For this review, take the finished solid that the model builds, in its own axes (mm). A direction names the side the tool comes from. Give positions to 0.01 mm unless a question says otherwise; leave off trailing zeros. Write each loop counter-clockwise with the first axis right and the second up, starting at its lowest first coordinate (ties: lowest second). Pieces come first, ordered by that corner, then holes. Notation, with made-up numbers: (-19, -36) -> (22, -36) arc R19 cw to (22, -28) -> close; hole circle Ø3 at (13, -5). An arc over 180 degrees is marked (long way). Answer as CSV lines item,"result".
Autodesk Inventor part; units mm, degrees
ref_plane "YZ Plane" through (0, 0, 0) normal (1, 0, 0) x (0, 1, 0)
ref_plane "XZ Plane" through (0, 0, 0) normal (0, 1, 0) x (-1, 0, 0)
ref_plane "XY Plane" through (0, 0, 0) normal (0, 0, 1) x (1, 0, 0)
sketch "スケッチ1" plane through (0, 0, 0) normal (1, 0, 0) x (0, 1, 0)
  line L0 (-114.0211, -198.214) -> (-114.0211, 205.786)
  line L1 (-114.0211, 122.786) -> (139.9789, 122.786)
  line L2 (139.9789, 122.786) -> (139.9789, 107.786)
  line L3 (139.9789, 107.786) -> (-114.0211, 107.786)
  line L4 (-114.0211, 107.786) -> (-114.0211, 122.786)
  line L5 (-74.0211, 147.286) -> (134.9789, 147.286)
  line L6 (134.9789, 147.286) -> (134.9789, -139.714)
  line L7 (134.9789, -139.714) -> (-74.0211, -139.714)
  line L8 (-74.0211, -139.714) -> (-74.0211, 147.286)
  line L9 (-134.0211, -198.214) -> (-134.0211, 205.786)
  line L10 (-134.0211, 3.786) -> (-114.0211, 3.786)
  line L11 (-114.0211, 205.786) -> (-134.0211, 205.786)
  line L12 (-114.0211, -115.214) -> (139.9789, -115.214)
  line L13 (139.9789, -100.214) -> (-114.0211, -100.214)
  line L14 (139.9789, -115.214) -> (139.9789, -100.214)
  line L15 (92.4789, 157.286) -> (82.4789, 157.286)
  line L16 (82.4789, 157.286) -> (82.4789, 3.786)
  line L17 (82.4789, 3.786) -> (92.4789, 3.786)
  line L18 (92.4789, 3.786) -> (92.4789, 157.286)
  line L19 (-21.5211, 157.286) -> (-31.5211, 157.286)
  line L20 (-31.5211, 157.286) -> (-31.5211, 3.786)
  line L21 (-31.5211, 3.786) -> (-21.5211, 3.786)
  line L22 (-21.5211, 3.786) -> (-21.5211, 157.286)
  line L23 (-114.0211, 135.286) -> (-134.0211, 135.286)
  line L24 (-84.0211, 122.786) -> (-84.0211, 107.786)
  circle A0 centre (-124.0211, 115.286) radius 1.5
  circle A1 centre (-124.0211, 125.286) radius 1.5
  line L25 (-114.0211, 135.286) -> (-114.0211, 122.786)
  line L26 (-114.0211, 107.786) -> (-134.0211, 107.786)
  line L27 (-134.0211, 135.286) -> (-134.0211, 107.786)
  circle A2 centre (-104.0211, 115.286) radius 1.5
  circle A3 centre (-94.0211, 115.286) radius 1.5
  line L28 (-84.0211, 107.786) -> (-64.0211, 107.786)
  line L29 (-64.0211, 107.786) -> (-64.0211, 101.786)
  line L30 (-64.0211, 101.786) -> (-84.0211, 101.786)
  line L31 (-84.0211, 101.786) -> (-84.0211, 107.786)
  line L32 (-31.5211, 157.286) -> (-37.5211, 157.286)
  line L33 (-37.5211, 157.286) -> (-37.5211, 137.286)
  line L34 (-37.5211, 137.286) -> (-31.5211, 137.286)
  line L35 (-31.5211, 137.286) -> (-31.5211, 157.286)
  line L36 (92.4789, 157.286) -> (98.4789, 157.286)
  line L37 (98.4789, 157.286) -> (98.4789, 137.286)
  line L38 (98.4789, 137.286) -> (92.4789, 137.286)
  line L39 (92.4789, 137.286) -> (92.4789, 157.286)
  line L40 (30.4789, 147.286) -> (30.4789, -139.714)
  line L41 (134.9789, 3.786) -> (-114.0211, 3.786)
  line L42 (-114.0211, 205.786) -> (-114.0211, -198.214)
  line L43 (-84.0211, -94.214) -> (-84.0211, -100.214)
  line L44 (-64.0211, -94.214) -> (-84.0211, -94.214)
  line L45 (-64.0211, -100.214) -> (-64.0211, -94.214)
  line L46 (-84.0211, -115.214) -> (-84.0211, -100.214)
  circle A4 centre (-94.0211, -107.714) radius 1.5
  circle A5 centre (-104.0211, -107.714) radius 1.5
  circle A6 centre (-124.0211, -107.714) radius 1.5
  circle A7 centre (-124.0211, -117.714) radius 1.5
  line L47 (-114.0211, -127.714) -> (-134.0211, -127.714)
  line L48 (-114.0211, -100.214) -> (-134.0211, -100.214)
  line L49 (-37.5211, -149.714) -> (-37.5211, -129.714)
  line L50 (-31.5211, -149.714) -> (-37.5211, -149.714)
  line L51 (-21.5211, -149.714) -> (-31.5211, -149.714)
  line L52 (-31.5211, -149.714) -> (-31.5211, 3.786)
  line L53 (-21.5211, 3.786) -> (-21.5211, -149.714)
  line L54 (-37.5211, -129.714) -> (-31.5211, -129.714)
  line L55 (82.4789, -149.714) -> (82.4789, 3.786)
  line L56 (92.4789, -149.714) -> (82.4789, -149.714)
  line L57 (92.4789, -149.714) -> (98.4789, -149.714)
  line L58 (98.4789, -149.714) -> (98.4789, -129.714)
  line L59 (98.4789, -129.714) -> (92.4789, -129.714)
  line L60 (92.4789, 3.786) -> (92.4789, -149.714)
  circle A8 centre (-26.5211, 115.286) radius 1.5
  circle A9 centre (87.4789, 115.286) radius 1.5
  circle A10 centre (87.4789, -107.714) radius 1.5
  circle A11 centre (-26.5211, -107.714) radius 1.5
  line L61 (-114.0211, 122.786) -> (-114.0211, 107.786)
  line L62 (-114.0211, -100.214) -> (-114.0211, -115.214)
  point P0 (0, 0)
  point P1 (-114.0211, 3.786)
  point P2 (-114.0211, 3.786)
  point P3 (-114.0211, 107.786)
  dimension "d0" = 15
  dimension "d1" = 287
  dimension "d2" = 209
  dimension "d3" = 83
  dimension "d4" = 10
  dimension "d5" = 10
  dimension "d6" = 30
  dimension "d7" = 3
  dimension "d8" = 7.5
  dimension "d9" = 10
  dimension "d10" = 3
  dimension "d11" = 10
  dimension "d12" = 10
  dimension "d13" = 10
  dimension "d14" = 3
  dimension "d15" = 3
  dimension "d16" = 10
  dimension "d17" = 10
  dimension "d18" = 7.5
  dimension "d19" = 7.5
  dimension "d20" = 6
  dimension "d21" = 10
  dimension "d22" = 10
  dimension "d23" = 5
  dimension "d24" = 143.5
  dimension "d25" = 10
  dimension "d26" = 6
  dimension "d27" = 20
  dimension "d28" = 10
  dimension "d29" = 6
  dimension "d30" = 20
  dimension "d31" = 0
  dimension "d32" = 0
  dimension "d33" = 52
  dimension "d34" = 52
  dimension "d35" = 3
  dimension "d36" = 3
  dimension "d37" = 5
  dimension "d38" = 7.5
  dimension "d39" = 7.5
  dimension "d40" = 5
extrude "押し出し1" add sketch "スケッチ1" against normal blind 2 contours L26 L9 L23 L0 | L0 L1 L24 L3
fillet "フィレット1" radius 2 6 edges at (-1, -84.0211, 122.786) (-1, -84.0211, 107.786) (-1, -114.0211, 122.786) (-1, -114.0211, 135.286) (-1, -134.0211, 135.286) (-1, -134.0211, 107.786)
equation "\"d13\" = d9"
equation "\"d17\" = d16"
equation "\"d19\" = d18"
equation "\"d34\" = d33"
properties part number "base_weel-v2-Plate-8" material "アルミニウム 6061"
Q1. Add section C-C (z = 114.25). Write out the cut boundary in (x, y).
Answer block:
outline,"(-2, -134.02) -> (0, -134.02) -> (0, -125.11) -> (-2, -125.11) -> close; (-2, -122.94) -> (0, -122.94) -> (0, -105.11) -> (-2, -105.11) -> close; (-2, -102.94) -> (0, -102.94) -> (0, -95.11) -> (-2, -95.11) -> close; (-2, -92.94) -> (0, -92.94) -> (0, -84.02) -> (-2, -84.02) -> close"
Q2. For faces 1 (the flat face through (0, -115, 119)), 2 (the flat face through (-1, -114.021, 129)), list the 3-axis set-ups (+Z, -Z, +X, -X, +Y, -Y) from which the entire face can be reached by the end or side of a thin tool; tool diameter is ignored.
Answer block:
face 1,"+Z, -Z, +X, +Y, -Y"
face 2,"+Z, +X, -X, +Y"
Q3. To check wall thickness, follow probe 1 along Z at (x, y) = (-1.7, -94); probe 2 along Y at (x, z) = (-0.55, 127.5); probe 3 along Y at (x, z) = (-0.65, 115.5). State the ranges of each line that lie inside material, in increasing order. Write a range as [from, to].
Answer block:
probe 1,"z = [107.79, 113.79], [116.79, 122.79]"
probe 2,"y = [-134.02, -114.02]"
probe 3,"y = [-134.02, -125.51], [-122.54, -105.51], [-102.54, -95.51], [-92.54, -84.02]"
Q4. Add section D-D (z = 126). Write out the cut boundary in (x, y).
Answer block:
outline,"(-2, -134.02) -> (0, -134.02) -> (0, -125.34) -> (-2, -125.34) -> close; (-2, -122.7) -> (0, -122.7) -> (0, -114.02) -> (-2, -114.02) -> close"
Q5. Add section B-B (y = -93.5). Write out the cut boundary in (x, z), plus the area to 3 significant figures.
Answer block:
outline,"(-2, 107.79) -> (0, 107.79) -> (0, 113.88) -> (-2, 113.88) -> close; (-2, 116.69) -> (0, 116.69) -> (0, 122.79) -> (-2, 122.79) -> close"
area,"24.4 mm2"
Q6. Draft analysis for pull direction Z (two halves, no side actions). For faces 3 (the cylindrical face through (-1.014, -113.42, 123.356)), 4 (the cylindrical face through (-1.014, -133.42, 108.356)), 5 (the flat face through (-1, -134.021, 121)), 6 (the cylindrical face through (-0.99, -93.21, 116.55)), state which applies: released by +Z, released by -Z, zero draft, split by the parting line, or undercut.
Answer block:
face 3,"released by +Z"
face 4,"released by -Z"
face 5,"zero draft"
face 6,"undercut"
Q7. Clearance check with flat-ended pins moving along their axes: pin 1 (4 mm diameter, centred on y = -94.02, z = 115.29, fed in from +X); pin 2 (1 mm diameter, centred on x = -1, y = -95.5, fed in from +Z). State where each tip first meets the part, or that it passes through.
Answer block:
pin 1,"stops at x = 0"
pin 2,"stops at z = 122.79"
Q8. Add section A-A (x = -1.5). Write out the cut boundary in (y, z), plus the area to 3 significant figures.
Answer block:
outline,"(-134.02, 109.79) arc R2 ccw to (-132.02, 107.79) -> (-86.02, 107.79) arc R2 ccw to (-84.02, 109.79) -> (-84.02, 120.79) arc R2 ccw to (-86.02, 122.79) -> (-112.02, 122.79) arc R2 cw to (-114.02, 124.79) -> (-114.02, 133.29) arc R2 ccw to (-116.02, 135.29) -> (-132.02, 135.29) arc R2 ccw to (-134.02, 133.29) -> close; hole circle Ø3 at (-124.02, 115.29); hole circle Ø3 at (-124.02, 125.29); hole circle Ø3 at (-104.02, 115.29); hole circle Ø3 at (-94.02, 115.29)"
area,"968 mm2"
